```python
from build123d import *

# Parameters (mm, degrees)
SKETCH1_R           = 2
BOSS_EXTRUDE1_DEPTH = 60
SKETCH2_W           = 8.571428572
SKETCH2_H           = 51.893398282
CUT_EXTRUDE1_DEPTH  = 8.5


with BuildPart() as part:
    # Sketch1 → Boss-Extrude1 (new body)
    with BuildSketch(Plane.XY):
        with BuildLine():
            Line((0, 0), (0, 51.893398282))
            Line((0, 51.893398282), (-27.651650429, 79.545048712))
            ThreePointArc((-27.651650429, 79.545048712), (-27.651650429, 84.848349571), (-22.348349571, 84.848349571))
            Line((-22.348349571, 84.848349571), (7.5, 55))
            Line((7.5, 55), (7.5, 0))
            Line((7.5, 0), (0, 0))
        make_face()
        with Locations((-25, 82.196699141)):
            Circle(SKETCH1_R, mode=Mode.SUBTRACT)
    extrude(amount=BOSS_EXTRUDE1_DEPTH)

    # Sketch2 → Cut-Extrude1 (cut, through all)
    with BuildSketch(Plane.ZY):
        with Locations((30, 25.946699141)):
            Rectangle(SKETCH2_W, SKETCH2_H)
        with Locations((47.142857143, 25.946699141)):
            Rectangle(SKETCH2_W, SKETCH2_H)
        with Locations((12.857142857, 25.946699141)):
            Rectangle(SKETCH2_W, SKETCH2_H)
    extrude(amount=-CUT_EXTRUDE1_DEPTH, mode=Mode.SUBTRACT)


solid = part.part
```
Could you check a few things on this model? Use its own coordinates, in mm. A direction names the side the tool comes from. Round coordinates to 2 decimals unless told otherwise and drop trailing zeros. Write each loop counter-clockwise with the first axis right and the second up, starting at its lowest first coordinate (ties: lowest second). Pieces come first, ordered by that corner, then holes. Notation, with made-up numbers: M 31.25,62 L 68.25,62 A31 cw 68.25,91 Z; hole C 64,-23.5 d8. An arc over 180 degrees is marked long. Write each question's results on one line, items separated by ' | '. Start each with the question number.
1. Imagine slicing it at C-C on x = 1.5. List the corners of the cut face in (y, z) for me.
2. I need wall thicknesses on L1, parallel to Z at x = 2, y = 50.5; L2, parallel to X at y = 81.5, z = 3.5; L3, parallel to X at y = 10.5, z = 42. Which ranges of each line are inside material? Lowest first, please. Write a range as from..to.
3. Imagine slicing it at B-B on x = -26. List the corners of the cut face in (y, z) for me.
4. Imagine slicing it at D-D on z = 9.5. List the corners of the cut face in (x, y) for me.
5. Thinking about a two-plate mould opening in Y: for faces 1 (the face through (4, 0, 39)), 2 (the face through (-7.6, 70.1, 29.6)), 3 (the face through (-27.7, 84.8, 29.6)), 4 (the face through (-25.26, 84.18, 29.58)), which applies, +Y half, -Y half, draft (parallel to the pull), parting line (faces both ways), or undercut?
6. On a 3-axis mill with a long thin cutter (end or side, diameter ignored), from which of +Z, -Z, +X, -X, +Y, -Y can I reach the whole of each face in a straight line? I mean faces 5 (the face through (0, 26, 4)), 6 (the face through (4, 0, 21)), 7 (the face through (4, 26, 42.857)). Say none if no direction works.
7. I'm going to push flat-ended pins straight in: pin 1 Ø8 at (x, z) = (-20, 8) entering from -Y; pin 2 Ø8 at (x, z) = (4, 12) entering from -Y; pin 3 Ø6 at (x, z) = (2, 48) entering from -Y; pin 4 Ø7 at (y, z) = (37.5, 39.5) entering from -X. Where does each tip first touch, or does it pass through?
8. Imagine slicing it at A-A on y = 16. List the corners of the cut face in (x, z) for me, and give its area (3 significant figures).
Result sheet:
1) outline: M 0,0 L 61,0 L 61,60 L 0,60 L 0,51.43 L 51.89,51.43 L 51.89,42.86 L 0,42.86 L 0,34.29 L 51.89,34.29 L 51.89,25.71 L 0,25.71 L 0,17.14 L 51.89,17.14 L 51.89,8.57 L 0,8.57 Z
2) L1: z = 0..8.57, 17.14..25.71, 34.29..42.86, 51.43..60 | L2: x = -28.68..-26.87, -23.13..-19 | L3: x = 0..7.5
3) outline: M 77.89,0 L 80.46,0 L 80.46,60 L 77.89,60 Z; M 83.93,0 L 85.81,0 L 85.81,60 L 83.93,60 Z
4) outline: M -27.65,79.55 L 0,51.89 L 7.5,51.89 L 7.5,55 L -22.35,84.85 A3.75 ccw Z; hole C -25,82.2 d4
5) face 1: -Y half | face 2: +Y half | face 3: parting line | face 4: undercut
6) face 5: +Z, -Z, -X, -Y | face 6: +Z, -Z, +X, -X, -Y | face 7: +X, -X, -Y
7) pin 1: stops at y = 67.89 | pin 2: stops at y = 0 | pin 3: stops at y = 51.89 | pin 4: stops at x = 0
8) outline: M 0,0 L 7.5,0 L 7.5,8.57 L 0,8.57 Z; M 0,17.14 L 7.5,17.14 L 7.5,25.71 L 0,25.71 Z; M 0,34.29 L 7.5,34.29 L 7.5,42.86 L 0,42.86 Z; M 0,51.43 L 7.5,51.43 L 7.5,60 L 0,60 Z | area: 257 mm^2
